Check sheet for the modelled part. Datum: model origin and axes. Units: mm. Face numbers are marked on the shaded views. A direction names the side the tool comes from. Round coordinates to 2 decimals unless told otherwise and drop trailing zeros. Order: outer loops, then holes, each group sorted by start corner. A loop starts at its lowest first (then second) coordinate and runs counter-clockwise, first axis right, second up.
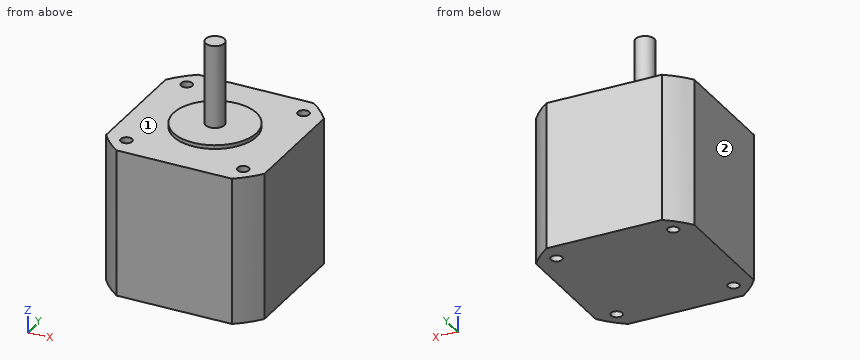
```python
from build123d import *

# Parameters (mm, degrees)
F0_R     = 1.5
F1_DEPTH = 39
F2_R     = 2.5
F3_DEPTH = 23
F4_R     = 11
F5_DEPTH = 1


with BuildPart() as f1:
    # F0 (on Top) → F1 (new body)
    with BuildSketch(Plane.XY):
        with BuildLine():
            ThreePointArc((-66.671558, -57.270136), (-64.056334, -60.325202), (-61.001267, -62.940426))
            Line((-61.001267, -62.940426), (-30.341848, -62.940426))
            ThreePointArc((-30.341848, -62.940426), (-27.286781, -60.325202), (-24.671558, -57.270136))
            Line((-24.671558, -57.270136), (-24.671558, -26.610716))
            ThreePointArc((-24.671558, -26.610716), (-27.286781, -23.55565), (-30.341848, -20.940426))
            Line((-30.341848, -20.940426), (-61.001267, -20.940426))
            ThreePointArc((-61.001267, -20.940426), (-64.056334, -23.55565), (-66.671558, -26.610716))
            Line((-66.671558, -26.610716), (-66.671558, -57.270136))
        make_face()
        with Locations((-61.171558, -57.440426)):
            Circle(F0_R, mode=Mode.SUBTRACT)
        with Locations((-30.171558, -57.440426)):
            Circle(F0_R, mode=Mode.SUBTRACT)
        with Locations((-61.171558, -26.440426)):
            Circle(F0_R, mode=Mode.SUBTRACT)
        with Locations((-30.171558, -26.440426)):
            Circle(F0_R, mode=Mode.SUBTRACT)
    extrude(amount=F1_DEPTH)

    # F2 (on face) → F3 (join)
    with BuildSketch(Plane.XY.offset(39)):
        with Locations((-45.671558, -41.940426)):
            Circle(F2_R)
    extrude(amount=F3_DEPTH)

    # F4 (on face) → F5 (join)
    with BuildSketch(Plane.XY.offset(39)):
        with Locations((-45.671558, -41.940426)):
            Circle(F4_R)
    extrude(amount=F5_DEPTH)


solid = f1.part
```
Item 1: Access from +Z, -Z, +X, -X, +Y, -Y to the whole of each face (thin tool, end or side, straight path). Record for the marked faces 1 and 2.
Answer:
face 1: +Z
face 2: +Z, -Z, -X, +Y, -Y
Item 2: Scan lines: line 1 along Y through (x, z) = (-31.5, 21); line 2 along X through (y, z) = (-27.5, 37); line 3 along Z through (x, y) = (-39, -41). Record each from-to range of solid material in increasing order.
Answer:
line 1: y = -62.94 to -58.14, -56.74 to -27.14, -25.74 to -20.94
line 2: x = -66.67 to -62.23, -60.11 to -31.23, -29.11 to -24.67
line 3: z = 0 to 40
Item 3: Sectioned sample at B-B (y = -32). Record the cut outline in (x, z).
Answer:
outline: (-66.67, 0) - (-24.67, 0) - (-24.67, 39) - (-40.96, 39) - (-40.96, 40) - (-50.38, 40) - (-50.38, 39) - (-66.67, 39) - close
Item 4: Go/stop test with flat-tipped pins: P1, Ø10, axis at x = -53, y = -36.5, coming from the +Z side; P2, Ø1.5, axis at x = -31, y = -33.5, coming from the +Z side; P3, Ø12, axis at y = -28.5, z = 49.5, coming from the +X side; P4, Ø3, axis at y = -43.5, z = 53.5, coming from the -X side. Record where each tip stops, or that it passes through.
Answer:
P1: stops at z = 40
P2: stops at z = 39
P3: passes through
P4: stops at x = -48.17
Item 5: Sectioned sample at A-A (z = 33). Record the cut outline in (x, y).
Answer:
outline: (-66.67, -57.27) arc R26 ccw to (-61, -62.94) - (-30.34, -62.94) arc R26 ccw to (-24.67, -57.27) - (-24.67, -26.61) arc R26 ccw to (-30.34, -20.94) - (-61, -20.94) arc R26 ccw to (-66.67, -26.61) - close; hole circle Ø3 at (-61.17, -57.44); hole circle Ø3 at (-61.17, -26.44); hole circle Ø3 at (-30.17, -57.44); hole circle Ø3 at (-30.17, -26.44)
Item 6: Sectioned sample at C-C (x = -46). Record the cut outline in (y, z), and give its area (3 significant figures).
Answer:
outline: (-62.94, 0) - (-20.94, 0) - (-20.94, 39) - (-30.95, 39) - (-30.95, 40) - (-39.46, 40) - (-39.46, 62) - (-44.42, 62) - (-44.42, 40) - (-52.94, 40) - (-52.94, 39) - (-62.94, 39) - close
area: 1,770 mm2
Item 7: Sectioned sample at D-D (x = -41). Record the cut outline in (y, z).
Answer:
outline: (-62.94, 0) - (-20.94, 0) - (-20.94, 39) - (-31.98, 39) - (-31.98, 40) - (-51.9, 40) - (-51.9, 39) - (-62.94, 39) - close
